Input: part model. Units: mm. Frame: model coordinates. A direction names the side the tool comes from. Coordinates: 2 decimals unless noted, no trailing zeros. Write each loop counter-clockwise with the first axis right and the second up, starting at its lowest first coordinate (ties: lowest second). Pieces come first, ordered by that corner, then holes. Notation, with made-up numbers: (33.25, 21) - (91.25, 21) arc R15 cw to (91.25, 26) - close; hole circle Ø8 at (-23, -29.5). An arc over 180 degrees is marked (long way). Use a Markdown table: item, result. Add a question column.
Q1. Section query C-C (z = 23.25). Return the cut outline in (x, y).
Q2. Section query D-D (x = 0). Return the cut outline in (y, z).
Q3. Section query B-B (x = 21.5). Return the cut outline in (y, z), then the cut area to 3 significant figures.
Q4. Material intervals for probe 1 along X at (y, z) = (-21, 24); probe 2 along Z at (x, y) = (21.5, -16.5); probe 3 along X at (y, z) = (8, 6.75), sorted ascending. Write a range as from..to.
Q5. Mould query, pull axis Y, two halves, no side actions, for faces 5 (the face through (-19, -6, 11)), 6 (the face through (-12.99, -6.76, 4.31)), 7 (the face through (24.247, -15.126, 8.879)). Classes: released by +Y, released by -Y, zero draft, split by the parting line, or undercut.
Q6. Pin query (flat end, axial travel): P1, Ø10.5, axis at x = 20.5, z = 10.5, coming from the +Y side; P2, Ø4, axis at x = -19, z = 9, coming from the +Y side; P3, Ø1.5, axis at x = -12, y = -6, coming from the -Z side; P4, Ø3, axis at x = -20, z = 20.5, coming from the +Y side. Return the tip coordinate at first contact, or that it passes through.
Q7. Section query A-A (y = -2). Return the cut outline in (x, z).
Q8. Set-up query: faces 1 (the face through (25.888, 9.21, 10.819)), 2 (the face through (13, 19, 8)), 3 (the face through (28, -6, 11)), 4 (the face through (-7, 9, 18)). Return all of +Z, -Z, +X, -X, +Y, -Y with unobstructed straight access to the full face (end or side cutting, diameter ignored); none if empty.
from build123d import *

# Parameters (mm, degrees)
SKETCH_1_W                   = 56
SKETCH_1_H                   = 48
EXTRUDE_1_DEPTH              = 18
SKETCH_9_R                   = 11
CUT_EXTRUDE_3_DEPTH          = 15
SKETCH_10_R                  = 8.5
CUT_EXTRUDE_4_DEPTH          = 17
HOLE_WIZARD_M3_2_D           = 2.5
HOLE_WIZARD_M3_2_DEPTH       = 8.5
HOLE_WIZARD_M3_2_TIP         = 0.751075774
HOLE_WIZARD_M5_1_D           = 5.5
HOLE_WIZARD_M5_1_CBORE_D     = 9.5
HOLE_WIZARD_M5_1_CBORE_DEPTH = 30
SKETCH_17_W                  = 56
SKETCH_17_H                  = 10
EXTRUDE_5_DEPTH              = 12
HOLE_WIZARD_5_5_5_5_1_D      = 5.5
SKETCH_21_R                  = 3
CUT_EXTRUDE_5_DEPTH          = 8


with BuildPart() as part:
    # 草图1 → 凸台-拉伸1 (new body)
    with BuildSketch(Plane.XY):
        Rectangle(SKETCH_1_W, SKETCH_1_H)
    extrude(amount=EXTRUDE_1_DEPTH)

    # 草图9 → 切除-拉伸3 (cut)
    with BuildSketch(Plane(origin=(0, 0, 0), x_dir=(-1, 0, 0), z_dir=(0, 0, -1))):
        with Locations((0, 1)):
            Circle(SKETCH_9_R)
    extrude(amount=-CUT_EXTRUDE_3_DEPTH, mode=Mode.SUBTRACT)

    # 草图10 → 切除-拉伸4 (cut)
    with BuildSketch(Plane(origin=(0, 0, 15), x_dir=(-1, 0, 0), z_dir=(0, 0, -1))):
        with Locations((0, 1)):
            Circle(SKETCH_10_R)
    extrude(amount=-CUT_EXTRUDE_4_DEPTH, mode=Mode.SUBTRACT)

    # M3 螺纹孔2
    with Locations(Plane(origin=(0, 0, 0), x_dir=(-1, 0, 0), z_dir=(0, 0, -1))):
        with Locations((12, 8), (-12, 8), (12, -6), (-12, -6)):
            Hole(HOLE_WIZARD_M3_2_D / 2, depth=HOLE_WIZARD_M3_2_DEPTH)
            with Locations((0, 0, -(HOLE_WIZARD_M3_2_DEPTH + HOLE_WIZARD_M3_2_TIP / 2))):  # 118° drill point
                Cone(0, HOLE_WIZARD_M3_2_D / 2, HOLE_WIZARD_M3_2_TIP, mode=Mode.SUBTRACT)

    # M5 六角头螺栓的柱形沉头孔1 (through all)
    with Locations(Plane(origin=(-28, 24, 18.039237195), x_dir=(1, 0, 0), z_dir=(0, 1, 0))):
        with Locations((6.5, 9.039237195), (49.5, 9.039237195)):
            CounterBoreHole(HOLE_WIZARD_M5_1_D / 2, HOLE_WIZARD_M5_1_CBORE_D / 2, HOLE_WIZARD_M5_1_CBORE_DEPTH)

    # 草图17 → 凸台-拉伸5 (add)
    with BuildSketch(Plane.XY.offset(18)):
        with Locations((0, -19)):
            Rectangle(SKETCH_17_W, SKETCH_17_H)
    extrude(amount=EXTRUDE_5_DEPTH)

    # Ø5.5 (5.5) 直径孔1 (through all)
    with Locations(Plane(origin=(0, -14, 0), x_dir=(1, 0, 0), z_dir=(0, 1, 0))):
        with Locations((-21.5, -24), (21.5, -24)):
            Hole(HOLE_WIZARD_5_5_5_5_1_D / 2)

    # 草图21 → 切除-拉伸5 (cut)
    with BuildSketch(Plane(origin=(0, 0, 0), x_dir=(-1, 0, 0), z_dir=(0, 0, -1))):
        with Locations((-12.5, 19)):
            Circle(SKETCH_21_R)
        with Locations((12.5, 19)):
            Circle(SKETCH_21_R)
    extrude(amount=-CUT_EXTRUDE_5_DEPTH, mode=Mode.SUBTRACT)


solid = part.part
Values follow:
| question | item | result |
|---|---|---|
| 1 | outline | (-28, -24) - (-24.15, -24) - (-24.15, -14) - (-28, -14) - close; (-18.85, -24) - (18.85, -24) - (18.85, -14) - (-18.85, -14) - close; (24.15, -24) - (28, -24) - (28, -14) - (24.15, -14) - close |
| 2 | outline | (-24, 0) - (-10, 0) - (-10, 15) - (-7.5, 15) - (-7.5, 18) - (-14, 18) - (-14, 30) - (-24, 30) - close; (9.5, 15) - (12, 15) - (12, 0) - (24, 0) - (24, 18) - (9.5, 18) - close |
| 3 | outline | (-24, 0) - (24, 0) - (24, 4.25) - (-6, 4.25) - (-6, 6.25) - (-24, 6.25) - close; (-24, 11.75) - (-6, 11.75) - (-6, 13.75) - (24, 13.75) - (24, 18) - (-14, 18) - (-14, 21.25) - (-24, 21.25) - close; (-24, 26.75) - (-14, 26.75) - (-14, 30) - (-24, 30) - close |
| 3 | area | 545 mm2 |
| 4 | probe 1 | -28..-24.25, -18.75..18.75, 24.25..28 |
| 4 | probe 2 | 0..6.25, 11.75..21.25, 26.75..30 |
| 4 | probe 3 | -28..-25.68, -17.32..-13.25, -10.75..-8.49, 8.49..10.75, 13.25..17.32, 25.68..28 |
| 5 | face 5 | released by +Y |
| 5 | face 6 | undercut |
| 5 | face 7 | zero draft |
| 6 | P1 | y = 24 |
| 6 | P2 | y = -6 |
| 6 | P3 | z = 8.8 |
| 6 | P4 | y = -14 |
| 7 | outline | (-28, 0) - (-10.58, 0) - (-10.58, 15) - (-7.95, 15) - (-7.95, 18) - (-28, 18) - close; (7.95, 15) - (10.58, 15) - (10.58, 0) - (28, 0) - (28, 18) - (7.95, 18) - close; hole circle Ø9.5 at (-21.5, 9); hole circle Ø9.5 at (21.5, 9) |
| 8 | face 1 | +Y |
| 8 | face 2 | -Z |
| 8 | face 3 | +Z, -Z, +X, +Y, -Y |
| 8 | face 4 | +Z, +X, -X, +Y |
